Design review of the part built by this model. Coordinates are the model's own, in mm. A direction names the side the tool comes from. Give positions to 0.01 mm unless a question says otherwise; leave off trailing zeros. Order: outer loops, then holes, each group sorted by start corner. A loop starts at its lowest first (then second) coordinate and runs counter-clockwise, first axis right, second up. Notation, with made-up numbers: (48, -4.75) -> (104, -4.75) arc R10 ccw to (104, 6.25) -> close; hole circle Ø11 at (-34, 0.25). An arc over 180 degrees is marked (long way). Use a Markdown table: item, result. Add a question column.
Autodesk Inventor part; units mm, degrees
ref_plane "YZ Plane" through (0, 0, 0) normal (1, 0, 0) x (0, 1, 0)
ref_plane "XZ Plane" through (0, 0, 0) normal (0, 1, 0) x (-1, 0, 0)
ref_plane "XY Plane" through (0, 0, 0) normal (0, 0, 1) x (1, 0, 0)
sketch "스케치1" plane through (0, 0, 0) normal (0, 0, 1) x (1, 0, 0)
  line L0 (-109.2986, 75.8401) -> (105.1639, 75.8401)
  line L1 (105.1639, 75.8401) -> (105.1639, -75.9568)
  line L2 (105.1639, -75.9568) -> (-109.2986, -75.9568)
  line L3 (-109.2986, -75.9568) -> (-109.2986, 75.8401)
  point P0 (0, 0)
extrude "돌출1" add sketch "스케치1" along normal blind 100
sketch "스케치2" plane through (0, 0, 100) normal (0, 0, 1) x (1, 0, 0)
  line L0 (-109.2986, -75.9568) -> (105.1639, -75.9568)
  line L1 (-26.2714, 75.9875) -> (105.1639, -75.9568)
  line L2 (105.1639, -75.9568) -> (105.1639, 75.9875)
  line L3 (105.1639, 75.9875) -> (-26.2714, 75.9875)
  point P0 (0, 0)
extrude "돌출2" cut sketch "스케치2" against normal blind 100
sketch "스케치3" plane through (-109.2986, 75.8401, 100) normal (0, 1, 0) x (1, 0, 0)
  point P0 (109.2986, 100)
sketch "스케치4" plane through (0, 0, 100) normal (0, 0, 1) x (1, 0, 0)
  line L0 (-109.2986, -75.9568) -> (-109.2986, 75.8401)
  line L1 (-109.2986, 75.8401) -> (-109.2986, -0.0583)
  line L2 (-26.1439, 75.8401) -> (105.1639, -75.9568)
  line L3 (39.51, -0.0583) -> (-26.1439, 75.8401)
  line L4 (-26.1439, 75.8401) -> (-109.2986, 75.8401)
  line L5 (-109.2986, -0.0583) -> (39.51, -0.0583)
  point P0 (0, 0)
extrude "돌출3" cut sketch "스케치4" against normal blind 50
sketch "스케치5" plane through (-109.2986, -0.0583, 100) normal (0, 1, 0) x (1, 0, 0)
  circle A0 centre (83.0272, 24.3451) radius 13.7114
  circle A1 centre (29.8194, 24.3451) radius 14.1089
  point P0 (109.2986, 100)
extrude "돌출4" cut sketch "스케치5" against normal blind 80
sketch "스케치6" plane through (105.1639, -75.9568, 100) normal (0.7563, 0.6542, 0) x (0, 0, -1)
  circle A0 centre (50, 0.3021) radius 21.6251
  point P0 (100, 126.2468)
extrude "돌출5" cut sketch "스케치6" against normal blind 80
properties part number "240510_3Dsketch01"
1) Add section B-B (z = 67.5). Give the boundary of the cut face in (x, y), then the cut area to 3 significant figures.
2) For L1, parallel to Y at x = 96, z = 89.5; L2, parallel to Y at x = 6, z = 90.5; L3, parallel to X at y = -17, z = 71, list the stretches that pass through material, from the lowest coordinate up. Write a range as [from, to].
3) The part is to be moulded in two halves that separate along Z. For faces 1 (the flat face through (-27, -37, 100)), 2 (the flat face through (-68, 75.84, 25)), 3 (the cylindrical face through (83.48, -65.73, 49.52)), say which applies: +Z half, -Z half, draft (parallel to the pull), parting line (faces both ways), or undercut.
4) Machinability: for faces 4 (the flat face through (-1, -75.957, 49)), 5 (the flat face through (-36, -0.058, 64)), which of the approach directions +Z, -Z, +X, -X, +Y, -Y give a long, thin tool a straight path to every point of the face, cutting with its end or side? Answer none if there is none.
5) Insertion check: pin 1 (10 mm diameter, centred on x = -34, y = 3.5, fed in from -Z); pin 2 (8 mm diameter, centred on x = 68, z = 68, fed in from +Y); pin 3 (2 mm diameter, centred on y = -31, z = 37, fed in from +X). Each pin has a flat end and moves straight along its axis. Give the tip position at first contact, or say it passes through.
6) Add section A-A (x = -75.5). Give the boundary of the cut face in (y, z), then the cut area to 3 significant figures.
7) Add section D-D (z = 7). Give the boundary of the cut face in (x, y).
8) Add section C-C (y = -57). Give the boundary of the cut face in (x, z).
Worked answers:
| question | item | result |
|---|---|---|
| 1 | outline | (-109.3, -75.96) -> (-90.99, -75.96) -> (-90.99, -0.06) -> (-109.3, -0.06) -> close; (-67.97, -75.96) -> (-37.29, -75.96) -> (-37.29, -0.06) -> (-67.97, -0.06) -> close; (-15.25, -75.96) -> (85.28, -75.96) -> (96.65, -66.12) -> (39.51, -0.06) -> (-15.25, -0.06) -> close |
| 1 | area | 10,300 mm^2 |
| 2 | L1 | [-75.96, -65.36] |
| 2 | L2 | [-75.96, -0.06] |
| 2 | L3 | [-109.3, -92.8], [-66.16, -39.17], [-13.37, 54.16] |
| 3 | face 1 | +Z half |
| 3 | face 2 | draft |
| 3 | face 3 | undercut |
| 4 | face 4 | +Z, -Z, +X, -X, -Y |
| 4 | face 5 | +Z, +X, -X, +Y |
| 5 | pin 1 | z = 0 |
| 5 | pin 2 | y = -28.37 |
| 5 | pin 3 | x = 67.14 |
| 6 | outline | (-75.96, 0) -> (75.84, 0) -> (75.84, 50) -> (-0.06, 50) -> (-0.06, 62.12) -> (-75.96, 62.12) -> close; (-75.96, 89.19) -> (-0.06, 89.19) -> (-0.06, 100) -> (-75.96, 100) -> close |
| 6 | area | 9,330 mm^2 |
| 7 | outline | (-109.3, -75.96) -> (105.16, -75.96) -> (-26.14, 75.84) -> (-109.3, 75.84) -> close |
| 8 | outline | (-109.3, 0) -> (88.77, 0) -> (88.77, 100) -> (-109.3, 100) -> close; hole circle Ø28.22 at (-79.48, 75.65); hole circle Ø27.42 at (-26.27, 75.65) |
